from build123d import *

# Parameters (mm, degrees)
BOSS_EXTRUDE1_DEPTH = 3
SKETCH2_W           = 78
SKETCH2_H           = 45
CUT_EXTRUDE1_DEPTH  = 10
FILLET1_R           = 10
CUT_EXTRUDE2_DEPTH  = 10
SKETCH4_W           = 16.5
SKETCH4_H           = 134.835477832
SKETCH4_H_2         = 126.10677569
BOSS_EXTRUDE2_DEPTH = 3
FILLET2_R           = 10
FILLET3_R           = 10


with BuildPart() as part:
    # Sketch1 → Boss-Extrude1 (new body)
    with BuildSketch(Plane(origin=(0, 0, 0), x_dir=(1, 0, 0), z_dir=(0, 1, 0))):
        Polygon((0, 0), (0, 75.000000004), (300, 65), (300, 0), align=None)
    boss_extrude1 = extrude(amount=BOSS_EXTRUDE1_DEPTH)

    # Mirror1: Boss-Extrude1 across Front Plane
    add(boss_extrude1.mirror(Plane.XY))

    # Sketch2 → Cut-Extrude1 (cut)
    with BuildSketch(Plane(origin=(0, 3, 0), x_dir=(1, 0, 0), z_dir=(0, 1, 0))):
        with Locations((55.5, 0)):
            Rectangle(SKETCH2_W, SKETCH2_H)
        with Locations((150, 0)):
            Rectangle(SKETCH2_W, SKETCH2_H)
        with Locations((244.5, 0)):
            Rectangle(SKETCH2_W, SKETCH2_H)
    extrude(amount=-CUT_EXTRUDE1_DEPTH, mode=Mode.SUBTRACT)

    # Fillet1
    fillet1_edges = [part.edges().sort_by_distance(p)[0] for p in [
        (16.5, 1.5, 22.5),
        (16.5, 1.5, -22.5),
        (94.5, 1.5, -22.5),
        (94.5, 1.5, 22.5),
        (111, 1.5, 22.5),
        (111, 1.5, -22.5),
        (189, 1.5, -22.5),
        (189, 1.5, 22.5),
        (205.5, 1.5, 22.5),
        (205.5, 1.5, -22.5),
        (283.5, 1.5, -22.5),
        (283.5, 1.5, 22.5),
    ]]
    fillet(fillet1_edges, radius=FILLET1_R)

    # Sketch3 → Cut-Extrude2 (cut)
    with BuildSketch(Plane(origin=(0, 3, 0), x_dir=(1, 0, 0), z_dir=(0, 1, 0))):
        with BuildLine():
            Line((12, 56.323336113), (12, 44))
            ThreePointArc((12, 44), (14.343145751, 38.343145751), (20, 36))
            Line((20, 36), (280, 36))
            ThreePointArc((280, 36), (285.656854249, 38.343145751), (288, 44))
            Line((288, 44), (288, 47.656669443))
            ThreePointArc((288, 47.656669443), (285.750310824, 53.218496969), (280.266518642, 55.652228699))
            Line((280.266518642, 55.652228699), (20.266518642, 64.318895369))
            ThreePointArc((20.266518642, 64.318895369), (14.438172474, 62.073646937), (12, 56.323336113))
        make_face()
    cut_extrude2 = extrude(amount=-CUT_EXTRUDE2_DEPTH, mode=Mode.SUBTRACT)

    # Mirror2: Cut-Extrude2 across plane
    add(cut_extrude2.mirror(Plane.XY), mode=Mode.SUBTRACT)

    # Sketch4 → Boss-Extrude2 (add)
    with BuildSketch(Plane(origin=(0, 3, 0), x_dir=(1, 0, 0), z_dir=(0, 1, 0))):
        with Locations((102.75, 0)):
            Rectangle(SKETCH4_W, SKETCH4_H)
        with Locations((197.25, 0)):
            Rectangle(SKETCH4_W, SKETCH4_H_2)
    extrude(amount=-BOSS_EXTRUDE2_DEPTH)

    # Fillet2
    fillet2_edges = [part.edges().sort_by_distance(p)[0] for p in [
        (111, 1.5, -36),
        (111, 1.5, -61.294445989),
        (94.5, 1.5, -36),
        (94.5, 1.5, -61.844445989),
        (189, 1.5, -36),
        (205.5, 1.5, -36),
        (205.5, 1.5, -58.144445988),
        (189, 1.5, -58.694445988),
    ]]
    fillet(fillet2_edges, radius=FILLET2_R)

    # Fillet3
    fillet3_edges = [part.edges().sort_by_distance(p)[0] for p in [
        (94.5, 1.5, 36),
        (111, 1.5, 36),
        (111, 1.5, 61.294445989),
        (94.5, 1.5, 61.844445989),
        (189, 1.5, 58.694445988),
        (189, 1.5, 36),
        (205.5, 1.5, 58.144445988),
        (205.5, 1.5, 36),
    ]]
    fillet(fillet3_edges, radius=FILLET3_R)


solid = part.part
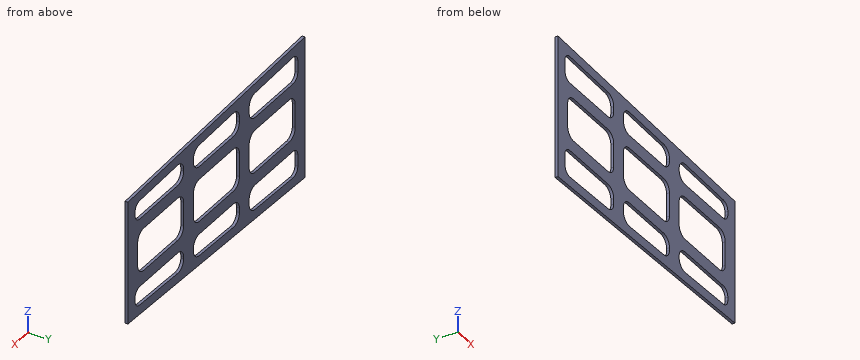
Build history of the part. All positions in model axes, mm. Round coordinates to 2 decimals unless told otherwise and drop trailing zeros. Loops run counter-clockwise (first coordinate to the right, second up) from the corner with the lowest first, then second, coordinate; pieces in that order, holes last. Notation, with made-up numbers: (88.5, 62) -> (141.5, 62) arc R28 cw to (141.5, 86) -> close; hole circle Ø5 at (22.25, 19). An arc over 180 degrees is marked (long way). Use CSV: the item, a comma, the result in double quotes. Start each with the question number.
Q1. Saw through at C-C on y = 1.45. Count the separate pieces of the cut face and the enclosed holes in it, and give its area (3 significant figures).
Q2. Flat gauge pins, fed straight in: pin 1 Ø1 at (x, y) = (118.5, 1.5) entering from -Z; pin 2 Ø1.5 at (x, y) = (248, 1) entering from +Z; pin 3 Ø1 at (x, y) = (56.5, 2) entering from +Z. Where does each tip first touch, or does it go through?
Q3. Drill centre lines: L1, parallel to X at y = 1.2, z = 2; L2, parallel to Z at x = 86.5, y = 1.25; L3, parallel to Z at x = 52, y = 1.3. Where is each one in solid material? Low to high.
Q4. Saw through at B-B on x = 170.5. Give the cut face in (y, z).
Q5. Saw through at A-A on z = 2. Give the cut face in (x, y).
Solutions:
1,separate pieces,"1"
1,enclosed holes,"9"
1,area,"20,500 mm^2"
2,pin 1,"stops at z = -71.07"
2,pin 2,"stops at z = 66.76"
2,pin 3,"stops at z = 73.13"
3,L1,"x = 0 to 16.5, 94.5 to 111, 189 to 205.5, 283.5 to 300"
3,L2,"z = -72.12 to -61.97, -36.2 to -22.3, 22.3 to 36.2, 61.97 to 72.12"
3,L3,"z = -73.27 to -63.26, -36 to -22.5, 22.5 to 36, 63.26 to 73.27"
4,outline,"(0, -69.32) -> (3, -69.32) -> (3, -59.31) -> (0, -59.31) -> close; (0, -36) -> (3, -36) -> (3, -22.5) -> (0, -22.5) -> close; (0, 22.5) -> (3, 22.5) -> (3, 36) -> (0, 36) -> close; (0, 59.31) -> (3, 59.31) -> (3, 69.32) -> (0, 69.32) -> close"
5,outline,"(0, 0) -> (16.5, 0) -> (16.5, 3) -> (0, 3) -> close; (94.5, 0) -> (111, 0) -> (111, 3) -> (94.5, 3) -> close; (189, 0) -> (205.5, 0) -> (205.5, 3) -> (189, 3) -> close; (283.5, 0) -> (300, 0) -> (300, 3) -> (283.5, 3) -> close"
